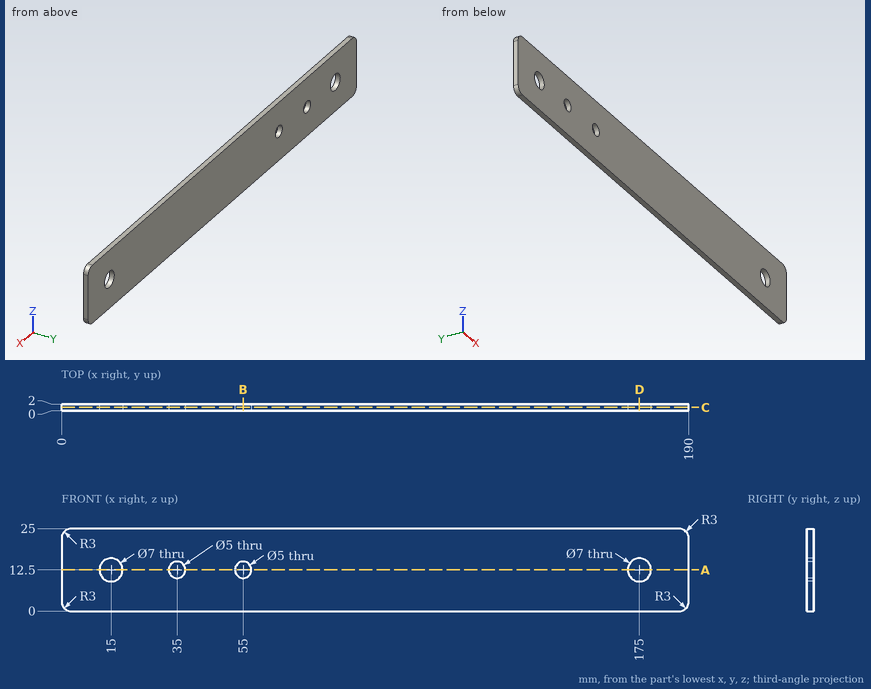
The drawing under review shows one solid part. Ordinate dimensions are in mm from its lowest x, y, z. Coordinates: 2 decimals unless noted, no trailing zeros. Loops run counter-clockwise (first coordinate to the right, second up) from the corner with the lowest first, then second, coordinate; pieces in that order, holes last. Notation, with made-up numbers: (-34.75, 53) - (-9.75, 53) arc R19 cw to (-9.75, 89) - close; hole circle Ø2 at (-33.75, 78). An arc over 180 degrees is marked (long way). Return JSON: item names as keys, results as strings.
Item 1: Take a section at A-A (z = 12.5). Give the boundary of the cut face in (x, y), then the cut area to 3 significant figures.
Determined:
{"outline": "(0, 0) - (11.5, 0) - (11.5, 2) - (0, 2) - close; (18.5, 0) - (32.5, 0) - (32.5, 2) - (18.5, 2) - close; (37.5, 0) - (52.5, 0) - (52.5, 2) - (37.5, 2) - close; (57.5, 0) - (171.5, 0) - (171.5, 2) - (57.5, 2) - close; (178.5, 0) - (190, 0) - (190, 2) - (178.5, 2) - close", "area": "332 mm2"}
Item 2: Take a section at D-D (x = 175). Give the boundary of the cut face in (y, z), then the cut area to 3 significant figures.
Determined:
{"outline": "(0, 0) - (2, 0) - (2, 9) - (0, 9) - close; (0, 16) - (2, 16) - (2, 25) - (0, 25) - close", "area": "36.0 mm2"}
Item 3: For line 1 (Z direction, x = 55, y = 1.45); line 2 (Z direction, x = 175, y = 1.5); line 3 (X direction, y = 1.35, z = 15.5), list the stretches that pass through material, from the lowest coordinate up.
Determined:
{"line 1": "z = 0 to 10, 15 to 25", "line 2": "z = 0 to 9, 16 to 25", "line 3": "x = 0 to 13.2, 16.8 to 173.2, 176.8 to 190"}
Item 4: Take a section at C-C (y = 1). Give the boundary of the cut face in (x, z).
Determined:
{"outline": "(0, 3) arc R3 ccw to (3, 0) - (187, 0) arc R3 ccw to (190, 3) - (190, 22) arc R3 ccw to (187, 25) - (3, 25) arc R3 ccw to (0, 22) - close; hole circle Ø7 at (15, 12.5); hole circle Ø5 at (35, 12.5); hole circle Ø5 at (55, 12.5); hole circle Ø7 at (175, 12.5)"}
Item 5: Take a section at B-B (x = 55). Give the boundary of the cut face in (y, z), then the cut area to 3 significant figures.
Determined:
{"outline": "(0, 0) - (2, 0) - (2, 10) - (0, 10) - close; (0, 15) - (2, 15) - (2, 25) - (0, 25) - close", "area": "40.0 mm2"}
